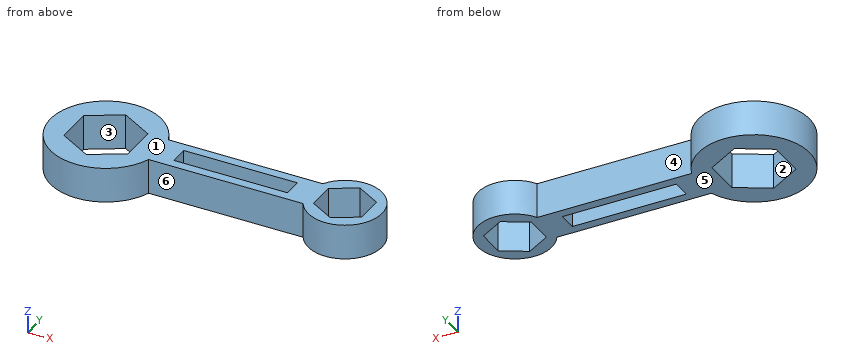
```python
from build123d import *

# Parameters (mm, degrees)
BOSS_EXTRUDE4_DEPTH = 19
SKETCH3_W           = 61.395220677
SKETCH3_H           = 10
CUT_EXTRUDE2_DEPTH  = 19


with BuildPart() as part:
    # Sketch1 → Boss-Extrude4 (new body)
    with BuildSketch(Plane.XY):
        with BuildLine():
            Line((-45.044820263, -26.313108204), (38.350400414, -26.313108204))
            ThreePointArc((38.350400414, -26.313108204), (75.67090849, -16.313108204), (38.350400414, -6.313108204))
            Line((38.350400414, -6.313108204), (-45.044820263, -6.313108204))
            ThreePointArc((-45.044820263, -6.313108204), (-103.32909151, -16.313108204), (-45.044820263, -26.313108204))
        make_face()
    extrude(amount=BOSS_EXTRUDE4_DEPTH)

    # Sketch3 → Cut-Extrude2 (cut)
    with BuildSketch(Plane.XY.offset(19)):
        Polygon((-73.32909151, 3.686891796), (-90.649599586, -6.313108204), (-90.649599586, -26.313108204), (-73.32909151, -36.313108204), (-56.008583435, -26.313108204), (-56.008583435, -6.313108204), align=None)
        Polygon((55.67090849, -1.313108204), (42.680527433, -8.813108204), (42.680527433, -23.813108204), (55.67090849, -31.313108204), (68.661289547, -23.813108204), (68.661289547, -8.813108204), align=None)
        with Locations((-3.347209925, -16.313108204)):
            Rectangle(SKETCH3_W, SKETCH3_H)
    extrude(amount=-CUT_EXTRUDE2_DEPTH, mode=Mode.SUBTRACT)


solid = part.part
```
Input: part model. Units: mm. Frame: model coordinates. Face numbers are marked on the shaded views. A direction names the side the tool comes from. Coordinates: 2 decimals unless noted, no trailing zeros. Loops run counter-clockwise (first coordinate to the right, second up) from the corner with the lowest first, then second, coordinate; pieces in that order, holes last. Notation, with made-up numbers: (59, 73) - (77, 73) arc R28 cw to (77, 103) - close; hole circle Ø10 at (-2, -28). An arc over 180 degrees is marked (long way). Answer in a Markdown table with one row per item.
(1) Pin query (flat end, axial travel): P1, Ø3, axis at y = -16, z = 10.5, coming from the -X side; P2, Ø11, axis at y = -14.5, z = 12, coming from the +X side; P3, Ø2, axis at x = -1, z = 14, coming from the +Y side. Return the tip coordinate at first contact, or that it passes through.
Model answer:
| item | result |
|---|---|
| P1 | stops at x = -103.33 |
| P2 | stops at x = 75.67 |
| P3 | stops at y = -6.31 |
(2) Material intervals for L1, parallel to X at y = -17, z = 9; L2, parallel to Y at x = 3.5, z = 8.75; L3, parallel to X at y = -3.5, z = 8.75, sorted ascending. Write a range as from..to.
Model answer:
| item | result |
|---|---|
| L1 | x = -103.32..-90.65, -56.01..-34.04, 27.35..42.68, 68.66..75.66 |
| L2 | y = -26.31..-21.31, -11.31..-6.31 |
| L3 | x = -100.46..-85.78, -60.88..-46.2, 40.31..51.88, 59.46..71.03 |
(3) Cut plane A-A on x = -15. Output: boundary loops of the cut face in (y, z), plus the area to 3 significant figures.
Model answer:
| item | result |
|---|---|
| outline | (-26.31, 0) - (-21.31, 0) - (-21.31, 19) - (-26.31, 19) - close; (-11.31, 0) - (-6.31, 0) - (-6.31, 19) - (-11.31, 19) - close |
| area | 190 mm² |
(4) Mould query, pull axis X, two halves, no side actions, for the marked faces 1 and 2. Classes: pulls with the +X half, pulls with the -X half, needs draft (parallel to the pull), parting line crosses it, or undercut.
Model answer:
| item | result |
|---|---|
| face 1 | needs draft |
| face 2 | undercut |
(5) Set-up query: the marked faces 3, 4, 5 and 6. Return all of +Z, -Z, +X, -X, +Y, -Y with unobstructed straight access to the full face (end or side cutting, diameter ignored); none if empty.
Model answer:
| item | result |
|---|---|
| face 3 | +Z, -Z |
| face 4 | +Z, -Z, +Y |
| face 5 | -Z, +X, -X, +Y, -Y |
| face 6 | +Z, -Z, -Y |
(6) Cut plane D-D on x = 65. Output: boundary loops of the cut face in (y, z), plus the area to 3 significant figures.
Model answer:
| item | result |
|---|---|
| outline | (-34, 0) - (-25.93, 0) - (-25.93, 19) - (-34, 19) - close; (-6.7, 0) - (1.38, 0) - (1.38, 19) - (-6.7, 19) - close |
| area | 307 mm² |
(7) Cut plane B-B on z = 14.5. Output: boundary loops of the cut face in (x, y).
Model answer:
| item | result |
|---|---|
| outline | (-45.04, -26.31) - (38.35, -26.31) arc R20 ccw (long way) to (38.35, -6.31) - (-45.04, -6.31) arc R30 ccw (long way) to start; hole (-90.65, -26.31) - (-73.33, -36.31) - (-56.01, -26.31) - (-56.01, -6.31) - (-73.33, 3.69) - (-90.65, -6.31) - close; hole (-34.04, -21.31) - (27.35, -21.31) - (27.35, -11.31) - (-34.04, -11.31) - close; hole (42.68, -23.81) - (55.67, -31.31) - (68.66, -23.81) - (68.66, -8.81) - (55.67, -1.31) - (42.68, -8.81) - close |
(8) Cut plane C-C on y = -29. Output: boundary loops of the cut face in (x, z), plus the area to 3 significant figures.
Model answer:
| item | result |
|---|---|
| outline | (-100.51, 0) - (-86, 0) - (-86, 19) - (-100.51, 19) - close; (-60.66, 0) - (-46.14, 0) - (-46.14, 19) - (-60.66, 19) - close; (40.21, 0) - (51.66, 0) - (51.66, 19) - (40.21, 19) - close; (59.68, 0) - (71.13, 0) - (71.13, 19) - (59.68, 19) - close |
| area | 987 mm² |
